Input: dimensioned drawing with shaded views. Units: mm. Origin: part minimum x, y, z. Give positions to 0.01 mm unless a question says otherwise; leave off trailing zeros. Loops run counter-clockwise (first coordinate to the right, second up) from the corner with the lowest first, then second, coordinate; pieces in that order, holes last. Notation, with made-up numbers: (-26, 88) -> (28, 88) arc R22 cw to (28, 104) -> close; hole circle Ø9 at (-16.5, -37.75). An arc over 180 degrees is marked (long way). Answer in a Markdown table with one row per item. Add a question column.
1) Section query B-B (y = 76.5). Return the cut outline in (x, z), plus the area to 3 significant figures.
2) First-contact query: P1, Ø2, axis at x = 1, z = 27.5, coming from the +Y side; P2, Ø3, axis at x = 3.5, z = 48, coming from the -Y side; P3, Ø2, axis at x = 3, y = 125.5, coming from the -Z side. Flat tips, straight axial feed; report the tip coordinate or a pass-through.
3) Line query: line 1 (Z direction, x = 4.5, y = 60); line 2 (Y direction, x = 1.5, z = 17); line 3 (Y direction, x = 4.75, z = 34). Output: solid intervals per line, ascending. Write a range as from..to.
4) Section query A-A (x = 5.25). Return the cut outline in (y, z) (1 decimal), plus the area to 3 significant figures.
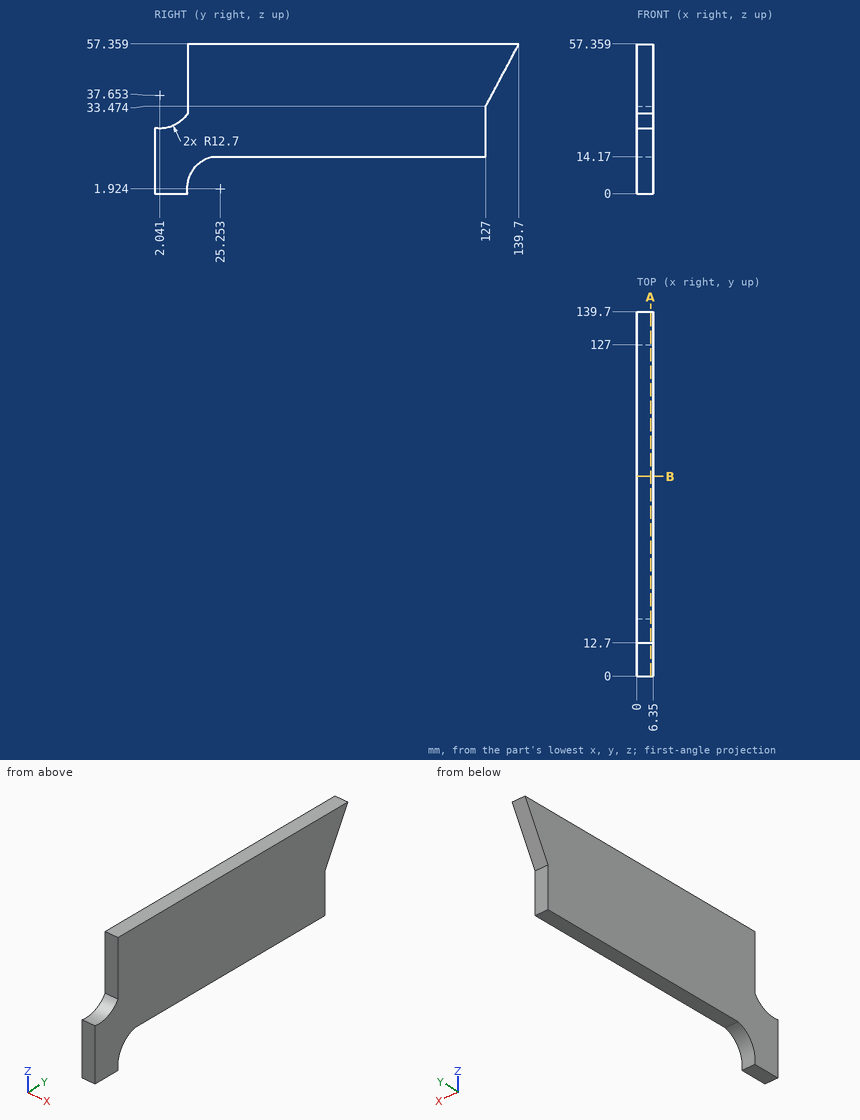
Evaluation:
| question | item | result |
|---|---|---|
| 1 | outline | (0, 14.17) -> (6.35, 14.17) -> (6.35, 57.36) -> (0, 57.36) -> close |
| 1 | area | 274 mm² |
| 2 | P1 | y = 127 |
| 2 | P2 | y = 12.7 |
| 2 | P3 | z = 14.17 |
| 3 | line 1 | 14.17..57.36 |
| 3 | line 2 | 0..127 |
| 3 | line 3 | 12.7..127.28 |
| 4 | outline | (0, 0) -> (12.7, 0) arc R12.7 cw to (21.9, 14.2) -> (127, 14.2) -> (127, 33.5) -> (139.7, 57.4) -> (12.7, 57.4) -> (12.7, 30.7) arc R12.7 cw to (0, 25.1) -> close |
| 4 | area | 5,450 mm² |
